from build123d import *

# Parameters (mm, degrees)
EXTRUDE_1_DEPTH          = 10
SKETCH_2_R               = 1.6
CUT_EXTRUDE_1_DEPTH      = 10
SKETCH_3_W               = 7
SKETCH_3_H               = 56
EXTRUDE_2_DEPTH          = 10
CUT_EXTRUDE_2_DEPTH      = 40.155628782
CUT_EXTRUDE_2_DEPTH_BACK = 40.155628782
SKETCH_4_R               = 1.6
SKETCH_5_W               = 20
SKETCH_5_H               = 56
EXTRUDE_3_DEPTH          = 10
SKETCH_6_R               = 1.6
CUT_EXTRUDE_3_DEPTH      = 40.155628782


with BuildPart() as part:
    # ｽｹｯﾁ1 → ﾎﾞｽ - 押し出し1 (new body)
    with BuildSketch(Plane.XY):
        Polygon((-60.928571429, 23.857142857), (-60.928571429, 16.857142857), (-40.928571429, 16.857142857), (-40.928571429, -25.142857143), (-60.928571429, -25.142857143), (-60.928571429, -32.142857143), (-33.928571429, -32.142857143), (-33.928571429, 23.857142857), align=None)
    extrude(amount=EXTRUDE_1_DEPTH)

    # ｽｹｯﾁ2 → ｶｯﾄ - 押し出し1 (cut)
    with BuildSketch(Plane(origin=(0, 0, 0), x_dir=(-1, 0, 0), z_dir=(0, 0, -1))):
        with Locations((45.928571429, 20.357142857)):
            Circle(SKETCH_2_R)
        with Locations((55.928571429, 20.357142857)):
            Circle(SKETCH_2_R)
        with Locations((45.928571429, -28.642857143)):
            Circle(SKETCH_2_R)
        with Locations((55.928571429, -28.642857143)):
            Circle(SKETCH_2_R)
    extrude(amount=-CUT_EXTRUDE_1_DEPTH, mode=Mode.SUBTRACT)

    # ｽｹｯﾁ3 → ﾎﾞｽ - 押し出し2 (add)
    with BuildSketch(Plane(origin=(0, 0, 0), x_dir=(-1, 0, 0), z_dir=(0, 0, -1))):
        with Locations((37.428571429, -4.142857143)):
            Rectangle(SKETCH_3_W, SKETCH_3_H)
    extrude(amount=EXTRUDE_2_DEPTH)

    # ｽｹｯﾁ4 → ｶｯﾄ - 押し出し2 (cut, two sides: drawn at the far end of the back side and taken through both)
    with BuildSketch(Plane.ZY.offset(40.928571429).offset(-CUT_EXTRUDE_2_DEPTH_BACK)):
        with Locations(Location((-5, 18.857142857, 0), (0, 0, 270))):
            Circle(SKETCH_4_R)
        with Locations(Location((-5, -27.142857143, 0), (0, 0, 270))):
            Circle(SKETCH_4_R)
    extrude(amount=CUT_EXTRUDE_2_DEPTH + CUT_EXTRUDE_2_DEPTH_BACK, mode=Mode.SUBTRACT)

    # ｽｹｯﾁ5 → ﾎﾞｽ - 押し出し3 (add)
    with BuildSketch(Plane(origin=(-33.928571429, 0, 0), x_dir=(0, 0, -1), z_dir=(1, 0, 0))):
        with Locations((0, -4.142857143)):
            Rectangle(SKETCH_5_W, SKETCH_5_H)
    extrude(amount=EXTRUDE_3_DEPTH)

    # ｽｹｯﾁ6 → ｶｯﾄ - 押し出し3 (cut, through all)
    with BuildSketch(Plane.ZY.offset(40.928571429)):
        with Locations(Location((-5, 18.857142857, 0), (0, 0, 270))):
            Circle(SKETCH_6_R)
        with Locations(Location((-5, -27.142857143, 0), (0, 0, 270))):
            Circle(SKETCH_6_R)
    extrude(amount=-CUT_EXTRUDE_3_DEPTH, mode=Mode.SUBTRACT)


solid = part.part
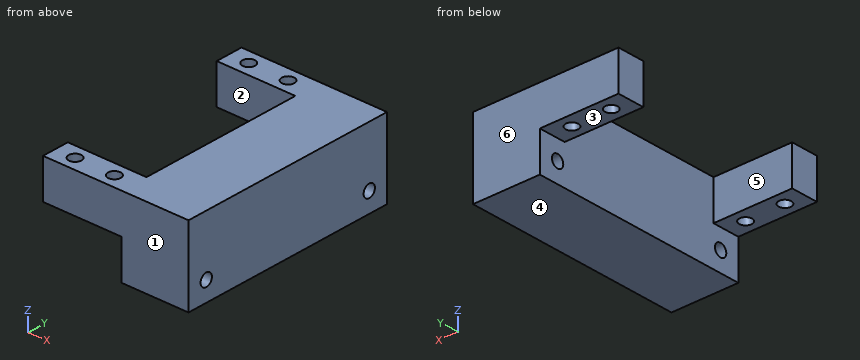
The listing builds one solid part. Answer for the finished solid, in the listing's coordinates (mm). Face numbers are marked on the shaded views. A direction names the side the tool comes from. Round coordinates to 2 decimals unless told otherwise and drop trailing zeros. Order: outer loops, then holes, each group sorted by start corner. A loop starts at its lowest first (then second) coordinate and runs counter-clockwise, first axis right, second up. Notation, with made-up numbers: (-11.75, 69.25) -> (14.25, 69.25) arc R11 cw to (14.25, 83.25) -> close; hole circle Ø4 at (-37.75, 85). An arc over 180 degrees is marked (long way). Put each result on its own line as item: value.
Q1. Determine the mould class of the marked faces 4, 5 and 6 for opening direction Y: pulls with the +Y half, pulls with the -Y half, needs draft (parallel to the pull), parting line crosses it, or undercut.
Results list:
face 4: needs draft
face 5: undercut
face 6: pulls with the +Y half
Q2. Section B-B, the plane z = -5 is taken. Write down the section's boundary in (x, y), and give its area (3 significant figures).
Results list:
outline: (-40.93, -32.14) -> (-23.93, -32.14) -> (-23.93, -28.74) -> (-40.93, -28.74) -> close; (-40.93, -25.54) -> (-23.93, -25.54) -> (-23.93, 17.26) -> (-40.93, 17.26) -> close; (-40.93, 20.46) -> (-23.93, 20.46) -> (-23.93, 23.86) -> (-40.93, 23.86) -> close
area: 843 mm^2
Q3. Consider line 1 along Y through (x, z) = (-28.5, -5); line 2 along Y through (x, z) = (-46.5, 4.5); line 3 along Y through (x, z) = (-50, 8.5). Determine where each line is inside the solid, lowest interval first.
Results list:
line 1: -32.14 to -28.74, -25.54 to 17.26, 20.46 to 23.86
line 2: -32.14 to -30.14, -27.15 to -25.14, 16.86 to 18.86, 21.85 to 23.86
line 3: -32.14 to -25.14, 16.86 to 23.86
Q4. Which of the six approach directions +Z, -Z, +X, -X, +Y, -Y give full straight-line access (tool end or side, diameter ignored) to the marked faces 1, 2 and 3?
Results list:
face 1: +Z, -Z, +X, -X, -Y
face 2: +Z, -Z, -X
face 3: -Z, -X, +Y, -Y
Q5. Section D-D, the plane y = 15 is taken. Write down the section's boundary in (x, z).
Results list:
outline: (-40.93, -10) -> (-23.93, -10) -> (-23.93, 10) -> (-40.93, 10) -> close
Q6. Section C-C, the plane x = -46 is taken. Write down the section's boundary in (y, z).
Results list:
outline: (-32.14, 0) -> (-30.24, 0) -> (-30.24, 10) -> (-32.14, 10) -> close; (-27.04, 0) -> (-25.14, 0) -> (-25.14, 10) -> (-27.04, 10) -> close; (16.86, 0) -> (18.76, 0) -> (18.76, 10) -> (16.86, 10) -> close; (21.96, 0) -> (23.86, 0) -> (23.86, 10) -> (21.96, 10) -> close
Q7. Section A-A, the plane x = -52 is taken. Write down the section's boundary in (y, z), and give its area (3 significant figures).
Results list:
outline: (-32.14, 0) -> (-25.14, 0) -> (-25.14, 10) -> (-32.14, 10) -> close; (16.86, 0) -> (23.86, 0) -> (23.86, 10) -> (16.86, 10) -> close
area: 140 mm^2
Q8. Each of these flat-tipped pins is pushed along its axis until it touches: P1, Ø1.9, axis at x = -45.93, y = 20.36, coming from the -Z side; P2, Ø12, axis at x = -53, z = -3.5, coming from the +Y side; P3, Ø2, axis at x = -51.5, y = 21.5, coming from the -Z side; P4, Ø8, axis at y = 1.5, z = 4.5, coming from the -X side. Where does it stop, or does it pass through?
Results list:
P1: through
P2: y = 23.86
P3: z = 0
P4: x = -40.93
